```python
from build123d import *

# Parameters (mm, degrees)
F1_DEPTH = 19.05
F2_W     = 47.8625434434
F2_H     = 13.97
F3_DEPTH = 60.96
F4_DEPTH = 6.35
F6_D     = 6.35
F8_DEPTH = 3.81


# Not quite as in the source:
# - a feature names something its author has since deleted; it is built from what else it names


with BuildPart() as f1:
    # F0 (on Top) → F1 (new body)
    with BuildSketch(Plane.XY):
        Polygon((-0.0274520135, 33.8990125982), (-26.4712717217, 33.8990125982), (-26.4712717217, -0.3909874018), (-26.4712717217, -34.6809874018), (16.3237974048, -34.6809874018), (26.8687282783, -34.6809874018), (26.8687282783, -0.3909874018), (26.8687282783, 33.8990125982), align=None)
    extrude(amount=-F1_DEPTH)

    # F2 (on face) → F3 (cut)
    with BuildSketch(Plane(origin=(0, 33.8990125982, 0), x_dir=(-1, 0, 0), z_dir=(0, 1, 0))):
        with Locations((0, -9.525)):
            Rectangle(F2_W, F2_H)
    extrude(amount=-F3_DEPTH, mode=Mode.SUBTRACT)

    # F0 (on Top) → F4 (join)
    with BuildSketch(Plane.XY):
        Polygon((-26.4712717217, -0.3909874018), (-26.4712717217, 33.8990125982), (-0.0274520135, 33.8990125982), (-0.0274520135, 37.7090125982), (-0.0274520135, 63.1090125982), (-38.1274520135, 63.1090125982), (-38.1274520135, -63.8909874018), (16.3237974048, -63.8909874018), (16.3237974048, -34.6809874018), (-26.4712717217, -34.6809874018), align=None)
        Polygon((-0.0274520135, 33.8990125982), (-26.4712717217, 33.8990125982), (-26.4712717217, -0.3909874018), (-26.4712717217, -34.6809874018), (16.3237974048, -34.6809874018), (26.8687282783, -34.6809874018), (26.8687282783, -0.3909874018), (26.8687282783, 33.8990125982), align=None)
        Polygon((-0.0274520135, 37.7090125982), (-0.0274520135, 33.8990125982), (26.8687282783, 33.8990125982), (26.8687282783, -0.3909874018), (38.0725479865, -0.3909874018), (38.0725479865, 63.1090125982), (-0.0274520135, 63.1090125982), align=None)
        Polygon((38.0725479865, -0.3909874018), (26.8687282783, -0.3909874018), (26.8687282783, -34.6809874018), (16.3237974048, -34.6809874018), (16.3237974048, -63.8909874018), (38.0725479865, -63.8909874018), align=None)
    extrude(amount=F4_DEPTH)

    # F6 (through all)
    with Locations(Plane.YZ.offset(26.8687282783)):
        with Locations((-15.6309874018, -9.525)):
            Hole(F6_D / 2)

    # F7 (on face) → F8 (cut)
    with BuildSketch(Plane.XY.offset(6.35)):
        Polygon((26.67, -34.29), (26.67, 0), (26.67, 34.29), (-26.67, 34.29), (-26.67, 0), (-26.67, -34.29), align=None)
    extrude(amount=-F8_DEPTH, mode=Mode.SUBTRACT)


solid = f1.part
```
Work out the finished part from the listing and answer in its coordinate system (mm). A direction names the side the tool comes from. Round coordinates to 2 decimals unless told otherwise and drop trailing zeros. Loops run counter-clockwise (first coordinate to the right, second up) from the corner with the lowest first, then second, coordinate; pieces in that order, holes last.
(1) Each of these flat-tipped pins is pushed along its axis until it touches: P1, Ø5, axis at x = 21.5, y = 10, coming from the +Z side; P2, Ø5.5, axis at y = -9, z = -13.5, coming from the +X side; P3, Ø4, axis at y = -15.63, z = -9.52, coming from the +X side; P4, Ø3, axis at x = 20, z = -6.5, coming from the +Y side. Where does it stop, or does it pass through?
Computed values:
P1: stops at z = 2.54
P2: stops at x = 26.87
P3: passes through
P4: stops at y = -27.06
(2) The mould has two halves that part along Y. Classify faces 1 (the flat face through (26.869, -1, -9)), 2 (the flat face through (2, 33.899, -17)), 3 (the flat face through (0, 34.29, 4)): pulls with the +Y half, pulls with the -Y half, needs draft (parallel to the pull), parting line crosses it, or undercut.
Computed values:
face 1: needs draft
face 2: pulls with the +Y half
face 3: undercut
(3) The part is cut by section B-B, the plane x = 14.5. Give the vertices of the cut face in (y, z).
Computed values:
outline: (-63.89, 0) - (-34.68, 0) - (-34.68, -19.05) - (33.9, -19.05) - (33.9, -16.51) - (-27.06, -16.51) - (-27.06, -2.54) - (33.9, -2.54) - (33.9, 0) - (63.11, 0) - (63.11, 6.35) - (34.29, 6.35) - (34.29, 2.54) - (-34.29, 2.54) - (-34.29, 6.35) - (-63.89, 6.35) - close
(4) The part is cut by section D-D, the plane z = -14. Give the vertices of the cut face in (x, y).
Computed values:
outline: (-26.47, -34.68) - (26.87, -34.68) - (26.87, 33.9) - (23.93, 33.9) - (23.93, -27.06) - (-23.93, -27.06) - (-23.93, 33.9) - (-26.47, 33.9) - close
(5) For faces 4 (the flat face through (0, 0, 2.54)), 5 (the flat face through (-26.471, 0, -9)), 6 (the flat face through (0, 4, -16.51)), determine the directions among +Z, -Z, +X, -X, +Y, -Y from which every point of the face is accessible in a straight line to the end or side of a thin tool.
Computed values:
face 4: +Z
face 5: -Z, -X, +Y, -Y
face 6: +Y
(6) The part is cut by section C-C, the plane y = 15. Give the vertices of the cut face in (x, z), and give its area (3 significant figures).
Computed values:
outline: (-38.13, 0) - (-26.47, 0) - (-26.47, -19.05) - (26.87, -19.05) - (26.87, 0) - (38.07, 0) - (38.07, 6.35) - (26.67, 6.35) - (26.67, 2.54) - (-26.67, 2.54) - (-26.67, 6.35) - (-38.13, 6.35) - close; hole (-23.93, -16.51) - (23.93, -16.51) - (23.93, -2.54) - (-23.93, -2.54) - close
area: 628 mm2
(7) The part is cut by section A-A, the plane z = 4.25. Give the vertices of the cut face in (x, y), and give its area (3 significant figures).
Computed values:
outline: (-38.13, -63.89) - (38.07, -63.89) - (38.07, 63.11) - (-38.13, 63.11) - close; hole (-26.67, -34.29) - (26.67, -34.29) - (26.67, 34.29) - (-26.67, 34.29) - close
area: 6,020 mm2
(8) Find the intervals of material crossed by L1, parallel to X at y = -17, z = -5.25; L2, parallel to Z at x = 19, y = 10; L3, parallel to Y at x = -24, z = 4.25, in increasing order.
Computed values:
L1: x = -26.47 to -23.93, 23.93 to 26.87
L2: z = -19.05 to -16.51, -2.54 to 2.54
L3: y = -63.89 to -34.29, 34.29 to 63.11
